Job drawing, mm, ordinate dimensions from the low corner. One solid piece. A direction names the side the tool comes from. Give positions to 0.01 mm unless a question says otherwise; leave off trailing zeros. Loops run counter-clockwise (first coordinate to the right, second up) from the corner with the lowest first, then second, coordinate; pieces in that order, holes last. Notation, with made-up numbers: M 8,46.5 L 21,46.5 A33 cw 21,77.5 Z; hole C 62,28.25 d8. An arc over 180 degrees is marked long. One line per question, with ' | ' between items.
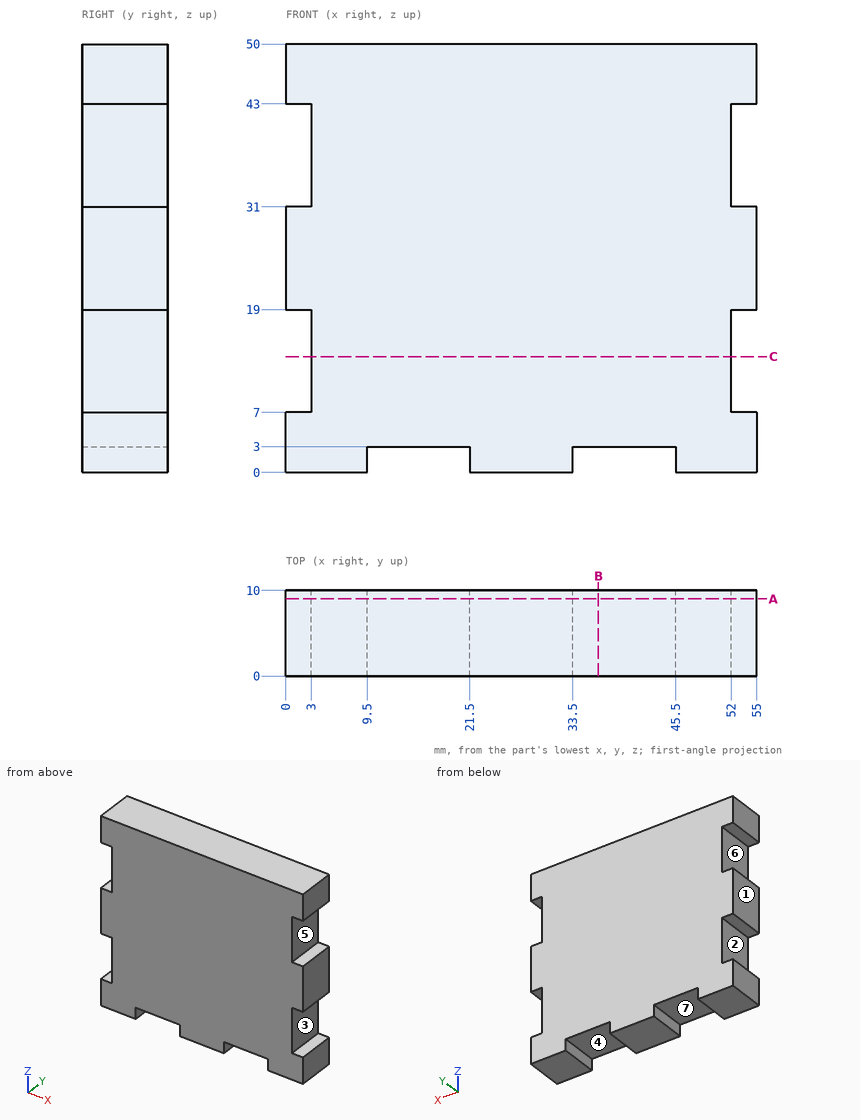
Item 1: Saw through at B-B on x = 36.5. Give the cut face in (y, z), and give its area (3 significant figures).
Conclusion:
outline: M 0,3 L 10,3 L 10,50 L 0,50 Z | area: 470 mm²
Item 2: Drop flat-ended pins along their axis: P1, Ø8, axis at x = 22, z = 5.5, coming from the -Y side; P2, Ø1.5, axis at y = 8.5, z = 39, coming from the -X side. Give the stop position or say it passes through.
Conclusion:
P1: y = 0 | P2: x = 3
Item 3: Mould opens along Z. For the marked faces 1, 2, 3 and 4 say: pulls with the +Z half, pulls with the -Z half, needs draft (parallel to the pull), parting line crosses it, or undercut.
Conclusion:
face 1: needs draft | face 2: undercut | face 3: undercut | face 4: pulls with the -Z half
Item 4: Drill centre lines: line 1 along Z through (x, y) = (53, 2.75); line 2 along X through (y, z) = (7.5, 36); line 3 along Z through (x, y) = (14, 7.75). Where is each one in solid material? Low to high. Write a range as [from, to].
Conclusion:
line 1: [0, 7], [19, 31], [43, 50] | line 2: [3, 52] | line 3: [3, 50]
Item 5: Saw through at C-C on z = 13.5. Give the cut face in (x, y), and give its area (3 significant figures).
Conclusion:
outline: M 3,0 L 52,0 L 52,10 L 3,10 Z | area: 490 mm²
Item 6: 3-axis set-ups, long thin cutter, end or side, ignore diameter. For the marked faces 5, 6 and 7: which of +Z, -Z, +X, -X, +Y, -Y reach the whole face in a straight line?
Conclusion:
face 5: +X, +Y, -Y | face 6: -X, +Y, -Y | face 7: -Z, +Y, -Y
Item 7: Saw through at A-A on y = 9. Give the cut face in (x, z), and give its area (3 significant figures).
Conclusion:
outline: M 0,0 L 9.5,0 L 9.5,3 L 21.5,3 L 21.5,0 L 33.5,0 L 33.5,3 L 45.5,3 L 45.5,0 L 55,0 L 55,7 L 52,7 L 52,19 L 55,19 L 55,31 L 52,31 L 52,43 L 55,43 L 55,50 L 0,50 L 0,43 L 3,43 L 3,31 L 0,31 L 0,19 L 3,19 L 3,7 L 0,7 Z | area: 2,530 mm²
